Geometry check sheet. Reference: the model listing, model coordinates, mm. A direction names the side the tool comes from. Coordinates: 2 decimals unless noted, no trailing zeros. Loops run counter-clockwise (first coordinate to the right, second up) from the corner with the lowest first, then second, coordinate; pieces in that order, holes last.
from build123d import *

# Parameters (mm, degrees)
BOSS_EXTRUDE1_DEPTH = 15
CUT_EXTRUDE1_DEPTH  = 5
CUT_EXTRUDE2_DEPTH  = 5
SKETCH4_R           = 0.75
CUT_EXTRUDE3_DEPTH  = 30
CUT_EXTRUDE4_DEPTH  = 5


with BuildPart() as part:
    # Sketch1 → Boss-Extrude1 (new body)
    with BuildSketch(Plane(origin=(0, 0, 0), x_dir=(1, 0, 0), z_dir=(0, 1, 0))):
        Polygon((0, 0), (-100, 0), (-130, 30), (0, 30), align=None)
    extrude(amount=BOSS_EXTRUDE1_DEPTH)

    # Sketch2 → Cut-Extrude1 (cut)
    with BuildSketch(Plane(origin=(0, 15, 0), x_dir=(1, 0, 0), z_dir=(0, 1, 0))):
        with BuildLine():
            Line((-135, 22.5), (-95, 22.5))
            ThreePointArc((-95, 22.5), (-87.5, 15), (-95, 7.5))
            Line((-95, 7.5), (-135, 7.5))
            ThreePointArc((-135, 7.5), (-142.5, 15), (-135, 22.5))
        make_face()
        with BuildLine():
            Line((20, 22.5), (-20, 22.5))
            ThreePointArc((-20, 22.5), (-27.5, 15), (-20, 7.5))
            Line((-20, 7.5), (20, 7.5))
            ThreePointArc((20, 7.5), (27.5, 15), (20, 22.5))
        make_face()
    extrude(amount=-CUT_EXTRUDE1_DEPTH, mode=Mode.SUBTRACT)

    # Sketch3 → Cut-Extrude2 (cut)
    with BuildSketch(Plane.XZ):
        with BuildLine():
            Line((0, -7.5), (0, -22.5))
            Line((0, -22.5), (-20, -22.5))
            ThreePointArc((-20, -22.5), (-27.5, -15), (-20, -7.5))
            Line((-20, -7.5), (0, -7.5))
        make_face()
        with BuildLine():
            Line((-122.5, -22.5), (-107.5, -7.5))
            Line((-107.5, -7.5), (-95, -7.5))
            ThreePointArc((-95, -7.5), (-87.5, -15), (-95, -22.5))
            Line((-95, -22.5), (-122.5, -22.5))
        make_face()
    extrude(amount=-CUT_EXTRUDE2_DEPTH, mode=Mode.SUBTRACT)

    # Sketch4 → Cut-Extrude3 (cut)
    with BuildSketch(Plane(origin=(0, 0, -30), x_dir=(-1, 0, 0), z_dir=(0, 0, -1))):
        with Locations((65, 7.5)):
            Circle(SKETCH4_R)
        with Locations((32.5, 7.5)):
            Circle(SKETCH4_R)
        with Locations((97.5, 7.5)):
            Circle(SKETCH4_R)
    extrude(amount=-CUT_EXTRUDE3_DEPTH, mode=Mode.SUBTRACT)

    # Sketch5 → Cut-Extrude4 (cut)
    with BuildSketch(Plane(origin=(0, 15, 0), x_dir=(1, 0, 0), z_dir=(0, 1, 0))):
        with BuildLine():
            Line((-77.5, 25), (-37.5, 25))
            ThreePointArc((-37.5, 25), (-33.964466094, 23.535533906), (-32.5, 20))
            Line((-32.5, 20), (-32.5, 10))
            ThreePointArc((-32.5, 10), (-33.964466094, 6.464466094), (-37.5, 5))
            Line((-37.5, 5), (-77.5, 5))
            ThreePointArc((-77.5, 5), (-81.035533906, 6.464466094), (-82.5, 10))
            Line((-82.5, 10), (-82.5, 20))
            ThreePointArc((-82.5, 20), (-81.035533906, 23.535533906), (-77.5, 25))
        make_face()
    extrude(amount=-CUT_EXTRUDE4_DEPTH, mode=Mode.SUBTRACT)


solid = part.part
(1) Sectioned sample at D-D on y = 13. Record the cut outline in (x, z), and give its area (3 significant figures).
Findings:
outline: (-130, -30) - (0, -30) - (0, -22.5) - (-20, -22.5) arc R7.5 cw to (-20, -7.5) - (0, -7.5) - (0, 0) - (-100, 0) - (-107.5, -7.5) - (-95, -7.5) arc R7.5 cw to (-95, -22.5) - (-122.5, -22.5) - close; hole (-82.5, -20) arc R5 ccw to (-77.5, -25) - (-37.5, -25) arc R5 ccw to (-32.5, -20) - (-32.5, -10) arc R5 ccw to (-37.5, -5) - (-77.5, -5) arc R5 ccw to (-82.5, -10) - close
area: 1,690 mm2
(2) Draft check along X on faces 6 (the cylindrical face through (-87.5, 2.46, -14.84)), 7 (the cylindrical face through (-27.5, 12.54, -15.16)), 8 (the cylindrical face through (-34, 12.54, -23.57)), 9 (the flat face through (-10, 2, -7.5)). Enter one of: +X half, -X half, draft (parallel to the pull), parting line (faces both ways), or undercut.
Findings:
face 6: -X half
face 7: +X half
face 8: undercut
face 9: draft
(3) Sectioned sample at B-B on y = 3.5. Record the cut outline in (x, z).
Findings:
outline: (-130, -30) - (0, -30) - (0, -22.5) - (-20, -22.5) arc R7.5 cw to (-20, -7.5) - (0, -7.5) - (0, 0) - (-100, 0) - (-107.5, -7.5) - (-95, -7.5) arc R7.5 cw to (-95, -22.5) - (-122.5, -22.5) - close
(4) Access from +Z, -Z, +X, -X, +Y, -Y to the whole of each face (thin tool, end or side, straight path). Record for faces 1 (the flat face through (-49, 7, 0)), 2 (the cylindrical face through (-33.93, 12.54, -6.5)), 3 (the flat face through (-101, 13, -7.5)), 4 (the flat face through (-10, 13, -22.5)), 5 (the flat face through (-109, 2, -22.5)).
Findings:
face 1: +Z, +X, -X, +Y, -Y
face 2: +Y
face 3: -X, +Y
face 4: +X, +Y
face 5: -X, -Y
(5) Scan lines: L1, parallel to Z at x = -47, y = 13.5; L2, parallel to Z at x = -94.5, y = 4.25; L3, parallel to Y at x = -65, z = -12. Record each from-to range of solid material in increasing order.
Findings:
L1: z = -30 to -25, -5 to 0
L2: z = -30 to -22.48, -7.52 to 0
L3: y = 0 to 6.75, 8.25 to 10
(6) Sectioned sample at A-A on z = -1.5. Record the cut outline in (x, y).
Findings:
outline: (-101.5, 0) - (0, 0) - (0, 15) - (-101.5, 15) - close; hole circle Ø1.5 at (-97.5, 7.5); hole circle Ø1.5 at (-65, 7.5); hole circle Ø1.5 at (-32.5, 7.5)
(7) Gauge pin test, flat ends, axial feed: pin 1 Ø12 at (x, z) = (-106, -14.5) entering from -Y; pin 2 Ø4 at (y, z) = (4, -18.5) entering from -X; pin 3 Ø1.5 at (y, z) = (12.5, -13.5) entering from -X. Record the tip position at first contact, or that the pin passes through.
Findings:
pin 1: stops at y = 5
pin 2: stops at x = -120.23
pin 3: stops at x = -87.85
(8) Sectioned sample at C-C on x = -57.5. Record the cut outline in (y, z).
Findings:
outline: (0, -30) - (15, -30) - (15, -25) - (10, -25) - (10, -5) - (15, -5) - (15, 0) - (0, 0) - close
